from build123d import *

# Parameters (mm, degrees)
EXTRUDE_1_DEPTH           = 8
HOLE_WIZARD_1_D           = 3.4
HOLE_WIZARD_1_DEPTH       = 10
HOLE_WIZARD_1_CSINK_D     = 6.5
HOLE_WIZARD_1_CSINK_ANGLE = 90
HOLE_WIZARD_1_TIP         = 1.021463052
FILLET_1_R                = 2
MM_2_D                    = 3
CHAMFER_1_SIZE            = 0.5
SKETCH_7_W                = 1
SKETCH_7_H                = 1.5
CUT_EXTRUDE_1_DEPTH       = 54.641089712


with BuildPart() as part:
    # 草图1 → 凸台-拉伸1 (new body)
    with BuildSketch(Plane.XY):
        with BuildLine():
            Line((-28.925442436, 34.47199994), (-23.783141558, 28.343644395))
            ThreePointArc((-23.783141558, 28.343644395), (0, 37), (23.783141558, 28.343644395))
            Line((23.783141558, 28.343644395), (28.925442436, 34.47199994))
            ThreePointArc((28.925442436, 34.47199994), (0, 45), (-28.925442436, 34.47199994))
        make_face()
    extrude(amount=EXTRUDE_1_DEPTH)

    # 打孔尺寸(%根据)内六角花形半沉头螺钉的类型1
    with Locations(Plane.XY.offset(8)):
        with Locations((0, 41)):
            CounterSinkHole(HOLE_WIZARD_1_D / 2, HOLE_WIZARD_1_CSINK_D / 2, depth=HOLE_WIZARD_1_DEPTH, counter_sink_angle=HOLE_WIZARD_1_CSINK_ANGLE)
            with Locations((0, 0, -(HOLE_WIZARD_1_DEPTH + HOLE_WIZARD_1_TIP / 2))):  # 118° drill point
                Cone(0, HOLE_WIZARD_1_D / 2, HOLE_WIZARD_1_TIP, mode=Mode.SUBTRACT)

    # 圆角1
    fillet_1_edges = [part.edges().sort_by_distance(p)[0] for p in [
        (-23.783141558, 28.343644395, 4),
        (-28.925442436, 34.47199994, 4),
        (28.925442436, 34.47199994, 4),
        (23.783141558, 28.343644395, 4),
    ]]
    fillet(fillet_1_edges, radius=FILLET_1_R)

    # 大小mm 暗销孔2 (through all)
    with Locations(Plane.XY.offset(8)):
        with Locations((20.406972636, 35.560588688), (-20.592886859, 35.453251061)):
            Hole(MM_2_D / 2)

    # 倒角1
    chamfer_1_edges = [part.edges().sort_by_distance(p)[0] for p in [
        (21.906972636, 35.560588688, 8),
        (-19.092886859, 35.453251061, 8),
    ]]
    chamfer(chamfer_1_edges, length=CHAMFER_1_SIZE)

    # 草图7 → 切除-拉伸1 (cut, through all)
    with BuildSketch(Plane.XY.offset(8)):
        with Locations((0, 45)):
            Rectangle(SKETCH_7_W, SKETCH_7_H)
    extrude(amount=-CUT_EXTRUDE_1_DEPTH, mode=Mode.SUBTRACT)


solid = part.part
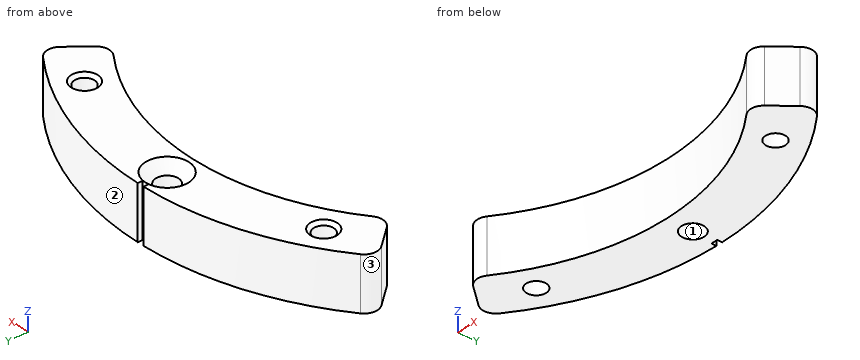
Check sheet for the modelled part. Datum: model origin and axes. Units: mm. Face numbers are marked on the shaded views. Give positions to 0.01 mm unless a question says otherwise; leave off trailing zeros. Loops run counter-clockwise (first coordinate to the right, second up) from the corner with the lowest first, then second, coordinate; pieces in that order, holes last. Notation, with made-up numbers: M 48.5,40 L 56.5,40 A22 ccw 56.5,64 Z; hole C 57.25,82 d4. An arc over 180 degrees is marked long. Answer as a JSON object with one key per item and string values. Group by question number.
Q1. Release check for a two-part mould opening along X. For the marked faces 1, 2 and 3 record: released by +X, released by -X, zero draft, split by the parting line, or undercut.
Q2. Cross-section at C-C on x = 9.5. Record the cut outline in (y, z), then the cut area to 3 significant figures.
Q3. Cross-section at A-A on y = 31.75. Record the cut outline in (x, z), then the cut area to 3 significant figures.
Q4. Material ranges on line 1 along Y through (x, z) = (19.5, 6.5); line 2 along X through (y, z) = (39.5, 6); line 3 along X through (y, z) = (41, 4), recorded low to high. Write a range as [from, to].
Q5. Cross-section at B-B on z = 3.5. Record the cut outline in (x, y), then the cut area to 3 significant figures.
Q6. Go/stop test with flat-tipped pins: P1, Ø4, axis at x = 20.41, y = 35.56, coming from the -Z side; P2, Ø3, axis at y = 41.5, z = 2, coming from the -X side; P3, Ø0.8, axis at x = 0, z = 2.5, coming from the +Y side; P4, Ø1.5, axis at x = 4, z = 4, coming from the -Y side. Record where each tip stops, or that it passes through.
Evaluation:
{
 "1": {"face 1": "undercut", "face 2": "released by +X", "face 3": "released by -X"},
 "2": {"outline": "M 35.76,0 L 43.99,0 L 43.99,8 L 35.76,8 Z", "area": "65.8 mm2"},
 "3": {"outline": "M -26.64,0 L -19,0 L -19,8 L -26.64,8 Z; M 19,0 L 26.64,0 L 26.64,8 L 19,8 Z", "area": "122 mm2"},
 "4": {"line 1": "y = [31.44, 34.37], [36.76, 40.56]", "line 2": "x = [-21.56, -0.8], [0.8, 21.56]", "line 3": "x = [-18.55, -1.7], [1.7, 18.55]"},
 "5": {"outline": "M -27.61,32.9 L -25.04,29.84 A2 ccw -22.3,29.53 A37 cw 22.3,29.53 A2 ccw 25.04,29.84 L 27.61,32.9 A2 ccw 27.29,35.78 A45 ccw 0.5,45 L 0.5,44.25 L -0.5,44.25 L -0.5,45 A45 ccw -27.29,35.78 A2 ccw Z; hole C -20.59,35.45 d3; hole C 0,41 d3.4; hole C 20.41,35.56 d3", "area": "431 mm2"},
 "6": {"P1": "stops at z = 0", "P2": "stops at x = -20.62", "P3": "stops at y = 44.25", "P4": "stops at y = 36.69"}
}
